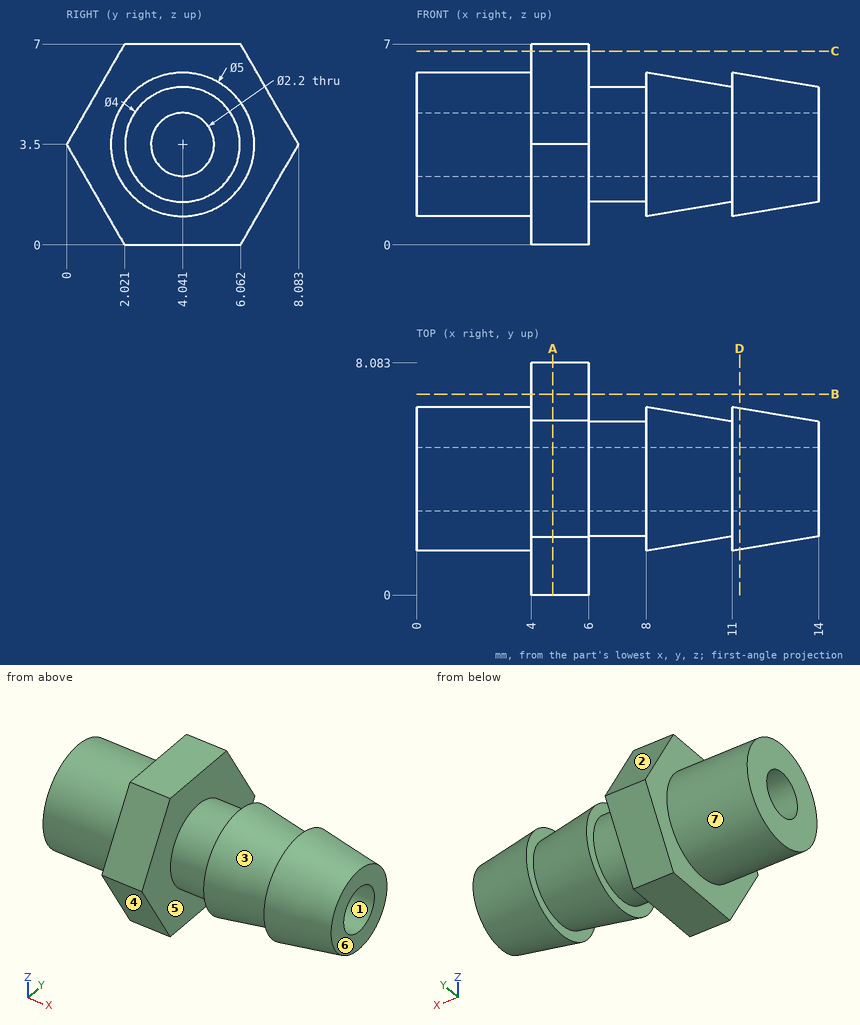
Design review of the part shown in the three views and the two pictorial views. Dimensions are in mm from the part's minimum x, y and z. A direction names the side the tool comes from. Round coordinates to 2 decimals unless told otherwise and drop trailing zeros. Loops run counter-clockwise (first coordinate to the right, second up) from the corner with the lowest first, then second, coordinate; pieces in that order, holes last. Notation, with made-up numbers: (84.25, 63.25) -> (121.25, 63.25) arc R18 cw to (121.25, 74.25) -> close; hole circle Ø7 at (22, 14). An arc over 180 degrees is marked (long way). Return JSON: item names as keys, results as strings.
(1) Add section C-C on z = 6.75. Write out the cut boundary in (x, y).
Solved:
{"outline": "(4, 1.88) -> (6, 1.88) -> (6, 6.21) -> (4, 6.21) -> close"}
(2) The part is to be moulded in two halves that separate along Z. For the marked faces 1, 2, 3 and 4, say which applies: released by +Z, released by -Z, zero draft, split by the parting line, or undercut.
Solved:
{"face 1": "undercut", "face 2": "released by +Z", "face 3": "split by the parting line", "face 4": "released by -Z"}
(3) For the marked faces 5, 6 and 7, list the 3-axis set-ups (+Z, -Z, +X, -X, +Y, -Y) from which the entire face can be reached by the end or side of a thin tool; tool diameter is ignored.
Solved:
{"face 5": "none", "face 6": "+Z, -Z, +X, +Y, -Y", "face 7": "-X"}
(4) Add section B-B on y = 7. Write out the cut boundary in (x, z) (1 decimal).
Solved:
{"outline": "(4, 1.6) -> (6, 1.6) -> (6, 5.4) -> (4, 5.4) -> close"}
(5) For pin 1 (1.5 mm diameter, centred on y = 4, z = 6, fed in from +X); pin 2 (1 mm diameter, centred on x = 1.5, y = 4, fed in from -Z); pin 3 (1.8 mm diameter, centred on y = 4.04, z = 3.5, fed in from -X), all flat-tipped, find the tip position at first contact; note any pin that passes through.
Solved:
{"pin 1": "x = 14", "pin 2": "z = 1", "pin 3": "through"}
(6) Add section D-D on x = 11.25. Write out the cut boundary in (y, z).
Solved:
{"outline": "circle Ø4.92 at (4.04, 3.5); hole circle Ø2.2 at (4.04, 3.5)"}
(7) Add section A-A on x = 4.75. Write out the cut boundary in (y, z).
Solved:
{"outline": "(0, 3.5) -> (2.02, 0) -> (6.06, 0) -> (8.08, 3.5) -> (6.06, 7) -> (2.02, 7) -> close; hole circle Ø2.2 at (4.04, 3.5)"}
(8) For line 1 (Y direction, x = 3.25, z = 3.5); line 2 (X direction, y = 3.25, z = 0.5); line 3 (Y direction, x = 9.75, z = 3.5), list the stretches that pass through material, from the lowest coordinate up.
Solved:
{"line 1": "1.54 to 2.94, 5.14 to 6.54", "line 2": "4 to 6", "line 3": "1.83 to 2.94, 5.14 to 6.25"}
